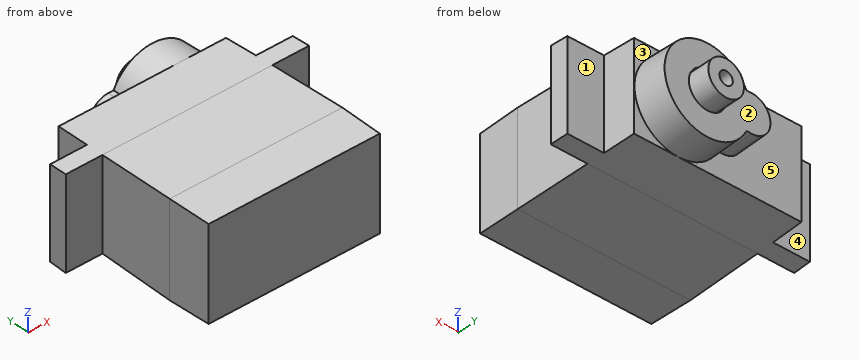
```python
from build123d import *

# Parameters (mm, degrees)
SKETCH8_W                 = 32.5
SKETCH8_H                 = 12.0777
BODY_MOUNTING_PLATE_DEPTH = 2.3749
SKETCH9_W                 = 22.6949
SKETCH9_H                 = 12.0777
BODY_TOP_DEPTH            = 4.318
BODY_TOP_DRAFT_1_5_ANGLE  = -1.5
SKETCH10_W                = 22.6949
SKETCH10_H                = 12.0777
BODY_MIDDLE_DEPTH         = 10.16
BODY_MIDDLE_DRAFT         = -1
SKETCH11_W                = 23.04958692
SKETCH11_H                = 12.43238692
BODY_BODOM_DEPTH          = 5.6515
BODY_BODOM_TAPER          = 1
BODY_TOPPER_DEPTH         = 4.3307
BODY_TOPPER_TAPER         = 1.5
SKETCH13_R                = 2.38125
SPINDLE_DEPTH             = 2.7432
SPINDLE_START             = -3.175
SKETCH18_R                = 2.50825
SKETCH18_R_2              = 2.38125
SPINDLE_OPENING_DEPTH     = 3.175
SKETCH14_R                = 0.889
SPINDLE_SCREW_HOLE_DEPTH  = 6.35


with BuildPart() as part:
    # Sketch8 → Body Mounting Plate (new body)
    with BuildSketch(Plane(origin=(0, 0, 0), x_dir=(1, 0, 0), z_dir=(0, 1, 0))):
        Rectangle(SKETCH8_W, SKETCH8_H)
    extrude(amount=BODY_MOUNTING_PLATE_DEPTH)

    # Sketch9 → Body Top (add)
    with BuildSketch(Plane(origin=(0, 2.3749, 0), x_dir=(1, 0, 0), z_dir=(0, 1, 0))):
        Rectangle(SKETCH9_W, SKETCH9_H)
    extrude(amount=BODY_TOP_DEPTH)

    # Body Top Draft 1.5
    body_top_draft_1_5_faces = [part.faces().sort_by_distance(p)[0] for p in [
        (11.34745, 4.5339, 0),
        (16.25, 1.18745, 0),
        (0, 3.059462209, -6.03885),
        (-11.34745, 4.5339, 0),
        (-16.25, 1.18745, 0),
        (0, 3.059462209, 6.03885),
    ]]
    draft(body_top_draft_1_5_faces, Plane(origin=(0, 0, 0), x_dir=(0, 0, -1), z_dir=(0, -1, 0)), BODY_TOP_DRAFT_1_5_ANGLE)


with BuildPart() as body_middle_tool:
    # Sketch10 → Body Middle (with draft: the straight prism first)
    with BuildSketch(Plane.XZ):
        Rectangle(SKETCH10_W, SKETCH10_H)
    extrude(amount=BODY_MIDDLE_DEPTH)
    # Body Middle: the draft: its side faces are tilted about the plane it starts from
    body_middle_sides = [body_middle_tool.faces().sort_by_distance(p)[0] for p in [
        (0, -5.08, 6.03885),
        (-11.34745, -5.08, 0),
        (0, -5.08, -6.03885),
        (11.34745, -5.08, 0),
    ]]
    draft(body_middle_sides, Plane.XZ, BODY_MIDDLE_DRAFT)


with BuildPart() as part_1:
    add(part.part)

    # Body Middle: add body_middle_tool
    add(body_middle_tool.part)

    # Sketch11 → Body Bodom (add)
    with BuildSketch(Plane.XZ.offset(10.16)):
        Rectangle(SKETCH11_W, SKETCH11_H)
    extrude(amount=BODY_BODOM_DEPTH, taper=BODY_BODOM_TAPER)

    # Sketch12 → Body Topper (add)
    with BuildSketch(Plane(origin=(0, 6.6929, 0), x_dir=(1, 0, 0), z_dir=(0, 1, 0))):
        with BuildLine():
            ThreePointArc((-0.652959754, 2.6035), (-3.256459754, 0), (-0.652959754, -2.6035))
            Line((-0.652959754, -2.6035), (-0.003901247, -2.6035))
            ThreePointArc((-0.003901247, -2.6035), (11.113590246, 0), (-0.003901247, 2.6035))
            Line((-0.003901247, 2.6035), (-0.652959754, 2.6035))
        make_face()
    extrude(amount=BODY_TOPPER_DEPTH, taper=BODY_TOPPER_TAPER)

    # Sketch13 → Spindle (add)
    with BuildSketch(Plane(origin=(0, 11.0236, 0), x_dir=(1, 0, 0), z_dir=(0, 1, 0))):
        with Locations(Location((5.25, 0, 0), (0, 0, 270))):
            Circle(SKETCH13_R)
    extrude(amount=SPINDLE_DEPTH)

    # Sketch18 → Spindle Opening (cut)
    with BuildSketch(Plane(origin=(0, 11.0236, 0), x_dir=(1, 0, 0), z_dir=(0, 1, 0)).offset(SPINDLE_START)):
        with Locations(Location((5.25, 0, 0), (0, 0, 270))):
            Circle(SKETCH18_R)
        with Locations(Location((5.25, 0, 0), (0, 0, 270))):
            Circle(SKETCH18_R_2, mode=Mode.SUBTRACT)
    extrude(amount=SPINDLE_OPENING_DEPTH, mode=Mode.SUBTRACT)

    # Sketch14 → Spindle Screw Hole (cut)
    with BuildSketch(Plane(origin=(0, 13.7668, 0), x_dir=(1, 0, 0), z_dir=(0, 1, 0))):
        with Locations(Location((5.25, 0, 0), (0, 0, 270))):
            Circle(SKETCH14_R)
    extrude(amount=-SPINDLE_SCREW_HOLE_DEPTH, mode=Mode.SUBTRACT)


solid = part_1.part
```
The model under review builds one solid part; all positions refer to its coordinate system, in mm. Face numbers are marked on the shaded views. A direction names the side the tool comes from. Round coordinates to 2 decimals unless told otherwise and drop trailing zeros. Loops run counter-clockwise (first coordinate to the right, second up) from the corner with the lowest first, then second, coordinate; pieces in that order, holes last.
1) Clearance check with flat-ended pins moving along their axes: P1, Ø2.5, axis at x = -14, z = -0.5, coming from the +Y side; P2, Ø3, axis at x = -5.5, z = -1, coming from the +Y side; P3, Ø0.9, axis at x = 5, z = 0, coming from the +Y side. State where each tip first meets the part, or that it passes through.
Values follow:
P1: stops at y = 2.37
P2: stops at y = 6.69
P3: stops at y = 7.42
2) Consider section B-B on x = 12. State the section outline as (y, z) points, then the cut area to 3 significant figures.
Values follow:
outline: (0, -6.04) - (2.37, -5.98) - (2.37, 5.98) - (0, 6.04) - close
area: 28.5 mm2
3) Consider section C-C on y = -2. State the section outline as (x, z) points.
Values follow:
outline: (-11.38, -6.07) - (11.38, -6.07) - (11.38, 6.07) - (-11.38, 6.07) - close
4) Tool access review of the marked faces 1, 2, 3, 4 and 5: name each direction out of +Z, -Z, +X, -X, +Y, -Y from which nothing blocks a thin tool from reaching the whole face with its end or side.
Values follow:
face 1: +Z, -Z, +X, +Y
face 2: +Y
face 3: +X, +Y
face 4: +Z, -Z, -X, +Y
face 5: -X, +Y
5) Wall thickness on line 1 along X through (y, z) = (10.25, 1.75); line 2 along X through (y, z) = (12.25, 0); line 3 along Y through (x, z) = (9, -4): over which ranges is each line inside the solid? List them lowest first.
Values follow:
line 1: x = -2.45 to 3.45, 3.64 to 6.86, 7.05 to 10.75
line 2: x = 2.87 to 4.36, 6.14 to 7.63
line 3: y = -15.81 to 11.02
6) Consider section A-A on y = 9.5. Give the number of separate pieces and of enclosed holes in the cut face, then the cut area to 3 significant figures.
Values follow:
separate pieces: 2
enclosed holes: 2
area: 112 mm2
